from build123d import *

# Parameters (mm, degrees)
SKETCH1_W          = 210
SKETCH1_H          = 210
MAINEXTRUDE_DEPTH  = 4
SKETCH1_6_R        = 1.5
SCREWHOLES_DEPTH   = 4
ROUNDEDCORNERS_R   = 10
SKETCH3_W          = 14
SKETCH3_H          = 14
SKETCH3_W_2        = 10
SKETCH3_H_2        = 150
CUTOUTS_DEPTH      = 10
SKETCH6_R          = 0.98
CUT_EXTRUDE1_DEPTH = 1


with BuildPart() as part:
    # Sketch1 → MainExtrude (new body)
    with BuildSketch(Plane(origin=(0, 0, 0), x_dir=(1, 0, 0), z_dir=(0, 1, 0))):
        Rectangle(SKETCH1_W, SKETCH1_H)
    extrude(amount=MAINEXTRUDE_DEPTH)

    # Sketch1<6> → ScrewHoles (cut)
    with BuildSketch(Plane(origin=(0, 0, 0), x_dir=(1, 0, 0), z_dir=(0, 1, 0))):
        with Locations((-99.833273811, 99.833273811)):
            Circle(SKETCH1_6_R)
        with Locations((-99.833273811, -99.833273811)):
            Circle(SKETCH1_6_R)
        with Locations((99.833273811, -99.833273811)):
            Circle(SKETCH1_6_R)
        with Locations((99.833273811, 99.833273811)):
            Circle(SKETCH1_6_R)
    extrude(amount=SCREWHOLES_DEPTH, mode=Mode.SUBTRACT)

    # RoundedCorners
    roundedcorners_edges = [part.edges().sort_by_distance(p)[0] for p in [
        (-105, 2, -105),
        (-105, 2, 105),
        (105, 2, 105),
        (105, 2, -105),
    ]]
    fillet(roundedcorners_edges, radius=ROUNDEDCORNERS_R)

    # Sketch3 → Cutouts (cut)
    with BuildSketch(Plane(origin=(0, 4, 0), x_dir=(1, 0, 0), z_dir=(0, 1, 0))):
        with Locations((-58.5, -78)):
            Rectangle(SKETCH3_W, SKETCH3_H)
        with Locations((-19.5, -78)):
            Rectangle(SKETCH3_W, SKETCH3_H)
        with Locations((19.5, -78)):
            Rectangle(SKETCH3_W, SKETCH3_H)
        with Locations((58.5, -78)):
            Rectangle(SKETCH3_W, SKETCH3_H)
        with Locations((-19.5, 17)):
            Rectangle(SKETCH3_W_2, SKETCH3_H_2)
        with Locations((-58.5, 17)):
            Rectangle(SKETCH3_W_2, SKETCH3_H_2)
        with Locations((19.5, 17)):
            Rectangle(SKETCH3_W_2, SKETCH3_H_2)
        with Locations((58.5, 17)):
            Rectangle(SKETCH3_W_2, SKETCH3_H_2)
    extrude(amount=-CUTOUTS_DEPTH, mode=Mode.SUBTRACT)

    # Sketch6 → Cut-Extrude1 (cut)
    with BuildSketch(Plane.XZ):
        with Locations((-70, 62)):
            Circle(SKETCH6_R)
        with Locations((70, 62)):
            Circle(SKETCH6_R)
        with Locations((70, -98)):
            Circle(SKETCH6_R)
        with Locations((-70, -98)):
            Circle(SKETCH6_R)
    extrude(amount=-CUT_EXTRUDE1_DEPTH, mode=Mode.SUBTRACT)


solid = part.part
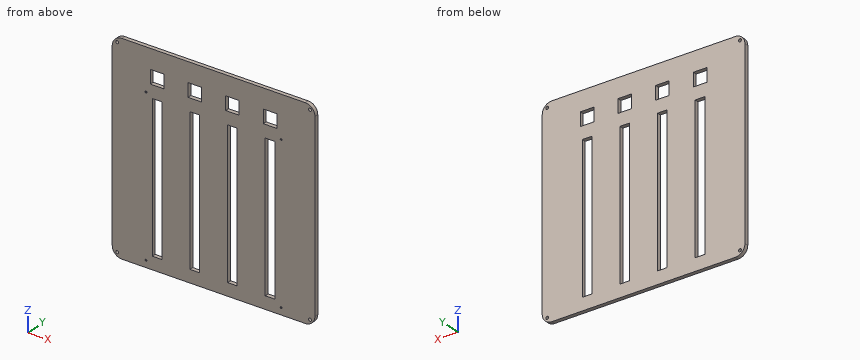
The listing builds one solid part. Answer for the finished solid, in the listing's coordinates (mm). Coordinates: 2 decimals unless noted, no trailing zeros. Loops run counter-clockwise (first coordinate to the right, second up) from the corner with the lowest first, then second, coordinate; pieces in that order, holes last. Notation, with made-up numbers: M 56.25,-20.5 L 101.25,-20.5 A17 ccw 101.25,-16.5 Z; hole C 76.25,-19.5 d6. An arc over 180 degrees is marked long. Answer in a Markdown table with one row per item.
1) Find section B-B (y = 1.9). Count the separate pieces of the cut face and the enclosed holes in it, then the cut area to 3 significant figures.
Answers below:
| item | result |
|---|---|
| separate pieces | 1 |
| enclosed holes | 12 |
| area | 37,200 mm^2 |
2) Find section A-A (z = -56.5). Determine the outline of the cut face in (x, y).
Answers below:
| item | result |
|---|---|
| outline | M -105,0 L -63.5,0 L -63.5,4 L -105,4 Z; M -53.5,0 L -24.5,0 L -24.5,4 L -53.5,4 Z; M -14.5,0 L 14.5,0 L 14.5,4 L -14.5,4 Z; M 24.5,0 L 53.5,0 L 53.5,4 L 24.5,4 Z; M 63.5,0 L 105,0 L 105,4 L 63.5,4 Z |
3) Given pin 1 (6 mm diameter, centred on x = -21, z = -40, fed in from +Y) (1 decimal), flat-ended and moving along its own axis, determine where the tip first touches the part or whether it passes through.
Answers below:
| item | result |
|---|---|
| pin 1 | through |
4) Find the intervals of material crossed by probe 1 along X at (y, z) = (0.75, -36.5); probe 2 along Z at (x, y) = (22.5, 2.2); probe 3 along Z at (x, y) = (70, 0.5), in increasing order.
Answers below:
| item | result |
|---|---|
| probe 1 | -105 to -63.5, -53.5 to -24.5, -14.5 to 14.5, 24.5 to 53.5, 63.5 to 105 |
| probe 2 | -105 to -92, 58 to 71, 85 to 105 |
| probe 3 | -105 to -98.98, -97.02 to 61.02, 62.98 to 105 |
